Autodesk Inventor part; units mm, degrees
ref_plane "swivel_to_body_XY" through (0, -3.2, 0) normal (0, 1, 0) x (1, 0, 0)
ref_plane "swivel_to_body_YZ" through (0, -3.2, 0) normal (1, 0, 0) x (0, 0, -1)
ref_plane "swivel_to_body_ZX" through (0, -3.2, 0) normal (0, 0, -1) x (0, 1, 0)
sketch "Sketch_1" plane through (0, 0, 0) normal (0, 1, 0) x (-1, 0, 0)
  arc A0 (80, 22.5) -> (73.5, 29) centre (73.5, 22.5) ccw
  line L0 (73.5, 29) -> (-73.5, 29)
  arc A1 (-73.5, 29) -> (-80, 22.5) centre (-73.5, 22.5) ccw
  line L1 (-80, 22.5) -> (-80, 17.8995)
  arc A2 (-80, 17.8995) -> (-77.9497, 12.9497) centre (-73, 17.8995) ccw
  line L2 (-77.9497, 12.9497) -> (-38.9289, -26.0711)
  arc A3 (-38.9289, -26.0711) -> (-31.8579, -29) centre (-31.8579, -19) ccw
  line L3 (-31.8579, -29) -> (31.8579, -29)
  arc A4 (31.8579, -29) -> (38.9289, -26.0711) centre (31.8579, -19) ccw
  line L4 (38.9289, -26.0711) -> (77.9497, 12.9497)
  arc A5 (77.9497, 12.9497) -> (80, 17.8995) centre (73, 17.8995) ccw
  line L5 (80, 17.8995) -> (80, 22.5)
  circle A6 centre (-69.5, 21) radius 2.65
  circle A7 centre (-27.5, -21) radius 2.65
  circle A8 centre (27.5, -21) radius 2.65
  circle A9 centre (69.5, 21) radius 2.65
extrude "Extrusion1" add sketch "Sketch_1" along normal blind 3.2
sketch "Sketch_2" plane through (0, 0, 0) normal (0, 1, 0) x (-1, 0, 0)
  arc A0 (64.9121, 11.2258) -> (64.7093, 12.7964) centre (64.205, 11.9329) ccw
  arc A1 (60.0432, 20.0952) -> (64.7093, 12.7964) centre (69.5, 21) ccw
  arc A2 (60.0432, 20.0952) -> (59.0477, 21) centre (59.0477, 20) ccw
  line L0 (59.0477, 21) -> (27.5, 21)
  arc A3 (27.5, 21) -> (27.5, 19) centre (27.5, 20) ccw
  line L1 (27.5, 19) -> (55.5447, 19)
  arc A4 (58.8009, 16.7833) -> (55.5447, 19) centre (55.5447, 15.5) ccw
  arc A5 (58.8009, 16.7833) -> (60.4356, 13.9228) centre (69.5, 21) ccw
  arc A6 (60.1518, 9.2939) -> (60.4356, 13.9228) centre (57.6769, 11.7688) ccw
  line L2 (60.1518, 9.2939) -> (36.7378, -14.1201)
  arc A7 (36.7378, -14.1201) -> (38.152, -15.5343) centre (37.4449, -14.8272) ccw
  line L3 (38.152, -15.5343) -> (64.9121, 11.2258)
extrude "Extrusion2" add sketch "Sketch_2" against normal blind 3.2
sketch "Sketch_3" plane through (0, 0, 0) normal (0, 1, 0) x (-1, 0, 0)
  arc A0 (-27.5, 19) -> (-27.5, 21) centre (-27.5, 20) ccw
  line L0 (-27.5, 21) -> (-59.0477, 21)
  arc A1 (-59.0477, 21) -> (-60.0432, 20.0952) centre (-59.0477, 20) ccw
  arc A2 (-64.7093, 12.7964) -> (-60.0432, 20.0952) centre (-69.5, 21) ccw
  arc A3 (-64.7093, 12.7964) -> (-64.9121, 11.2258) centre (-64.205, 11.9329) ccw
  line L1 (-64.9121, 11.2258) -> (-38.152, -15.5343)
  arc A4 (-38.152, -15.5343) -> (-36.7378, -14.1201) centre (-37.4449, -14.8272) ccw
  line L2 (-36.7378, -14.1201) -> (-60.1518, 9.2939)
  arc A5 (-60.4356, 13.9228) -> (-60.1518, 9.2939) centre (-57.6769, 11.7688) ccw
  arc A6 (-60.4356, 13.9228) -> (-58.8009, 16.7833) centre (-69.5, 21) ccw
  arc A7 (-55.5447, 19) -> (-58.8009, 16.7833) centre (-55.5447, 15.5) ccw
  line L3 (-55.5447, 19) -> (-27.5, 19)
extrude "Extrusion3" add sketch "Sketch_3" against normal blind 3.2
ref_plane "swivel_to_body_XY" through (0, -3.2, 0) normal (0, 1, 0) x (1, 0, 0)
ref_plane "swivel_to_body_YZ" through (0, -3.2, 0) normal (1, 0, 0) x (0, 0, -1)
ref_plane "swivel_to_body_ZX" through (0, -3.2, 0) normal (0, 0, -1) x (0, 1, 0)
ref_plane "swivel_to_dummy_XY" through (0, 3.2, 0) normal (0, -1, 0) x (1, 0, 0)
ref_plane "swivel_to_dummy_YZ" through (0, 3.2, 0) normal (1, 0, 0) x (0, 0, 1)
ref_plane "swivel_to_dummy_ZX" through (0, 3.2, 0) normal (0, 0, 1) x (0, -1, 0)
properties part number "SWIVEL-HSMCS50"
Design review of the part built by this model. Coordinates are the model's own, in mm. A direction names the side the tool comes from. Coordinates: 2 decimals unless noted, no trailing zeros. Write each loop counter-clockwise with the first axis right and the second up, starting at its lowest first coordinate (ties: lowest second). Pieces come first, ordered by that corner, then holes.
1) Add section C-C (x = -47). Write out the cut boundary in (y, z), plus the area to 3 significant figures.
2) Add section A-A (x = -69.5). Write out the cut boundary in (y, z).
3) Add section D-D (z = -12). Write out the cut boundary in (x, y).
4) Mouldability with a two-part tool opening along X and no side actions: class faces 1 (the cylindrical face through (61.53, -1.58, 15.83)), 2 (the flat face through (-51.345, -1.578, -2.342)), 3 (the flat face through (1, 3.2, 7)), 4 (the cylindrical face through (57.49, -1.58, 18.41)) as +X half, -X half, draft (parallel to the pull), parting line (faces both ways), or undercut.
5) Machinability: for faces 5 (the cylindrical face through (66.972, 1.578, 20.204)), 6 (the cylindrical face through (-79.5, 1.6, 15.3)), 7 (the cylindrical face through (-61.46, -1.58, 15.94)), 8 (the cylindrical face through (-61.17, -1.58, 11.52)), 9 (the flat face through (-43, -2, 21)), which of the approach directions +Z, -Z, +X, -X, +Y, -Y give a long, thin tool a straight path to every point of the face, cutting with its end or side? Answer none if there is none.
6) To check wall thickness, follow L1, parallel to X at y = 2, z = 20.5; L2, parallel to Y at x = 46, z = -1; L3, parallel to X at y = -1, z = 14. State the ranges of each line that lie inside material, in increasing order.
7) Insertion check: pin 1 (1.6 mm diameter, centred on x = 45.5, y = -1.5, fed in from -Z); pin 2 (17.5 mm diameter, centred on x = 12, z = -14.5, fed in from -Y); pin 3 (1.6 mm diameter, centred on x = 50, y = -1.5, fed in from +Z). Each pin has a flat end and moves straight along its axis. Give the tip position at first contact, or say it passes through.
8) Add section B-B (y = -1). Write out the cut boundary in (x, z), plus the area to 3 significant figures.
Check result:
1. outline: (-3.2, -6.69) - (0, -6.69) - (0, -18) - (3.2, -18) - (3.2, 29) - (0, 29) - (0, 21) - (-3.2, 21) - (-3.2, 19) - (0, 19) - (0, -3.86) - (-3.2, -3.86) - close
1. area: 166 mm2
2. outline: (0, 4.5) - (3.2, 4.5) - (3.2, 18.35) - (0, 18.35) - close; (0, 23.65) - (3.2, 23.65) - (3.2, 29) - (0, 29) - close
3. outline: (-53, 0) - (-41.69, 0) - (-41.69, -3.2) - (-38.86, -3.2) - (-38.86, 0) - (38.86, 0) - (38.86, -3.2) - (41.69, -3.2) - (41.69, 0) - (53, 0) - (53, 3.2) - (-53, 3.2) - close
4. face 1: +X half
4. face 2: -X half
4. face 3: draft
4. face 4: undercut
5. face 5: +Y, -Y
5. face 6: -Z, -X, +Y, -Y
5. face 7: +Z, -X, -Y
5. face 8: -Y
5. face 9: +Z, +X, -X, -Y
6. L1: x = -80 to -72.1, -66.9 to 66.9, 72.1 to 80
6. L2: y = 0 to 3.2
6. L3: x = -63.08 to -60.38, 60.38 to 63.08
7. pin 1: stops at z = -8.99
7. pin 2: stops at y = 0
7. pin 3: stops at z = 21
8. outline: (-64.91, 11.23) - (-38.15, -15.53) arc R1 ccw to (-36.74, -14.12) - (-60.15, 9.29) arc R3.5 cw to (-60.44, 13.92) arc R11.5 ccw to (-58.8, 16.78) arc R3.5 cw to (-55.54, 19) - (-27.5, 19) arc R1 ccw to (-27.5, 21) - (-59.05, 21) arc R1 ccw to (-60.04, 20.1) arc R9.5 cw to (-64.71, 12.8) arc R1 ccw to start; (27.5, 19) - (55.54, 19) arc R3.5 cw to (58.8, 16.78) arc R11.5 ccw to (60.44, 13.92) arc R3.5 cw to (60.15, 9.29) - (36.74, -14.12) arc R1 ccw to (38.15, -15.53) - (64.91, 11.23) arc R1 ccw to (64.71, 12.8) arc R9.5 cw to (60.04, 20.1) arc R1 ccw to (59.05, 21) - (27.5, 21) arc R1 ccw to start
8. area: 330 mm2
